Work out the finished part from the listing and answer in its coordinate system (mm). A direction names the side the tool comes from. Coordinates: 2 decimals unless noted, no trailing zeros. Order: outer loops, then holes, each group sorted by start corner. A loop starts at its lowest first (then second) coordinate and runs counter-clockwise, first axis right, second up. Notation, with made-up numbers: M 40.5,46 L 64.5,46 A13 cw 64.5,60 Z; hole C 74.25,-26.5 d7. An arc over 180 degrees is marked long. Use a Markdown table: item, result. Add a question column.
from build123d import *

# Parameters (mm, degrees)
F1_DEPTH  = 3
F2_R      = 1.5
F3_DEPTH  = 25
F5_DEPTH  = 3
F7_D      = 3
F7_DEPTH  = 3
F7_TIP    = 0.9012909285
F8_DEPTH  = 3
F9_R      = 1.5
F9_R_2    = 4
F10_DEPTH = 25


# Not quite as in the source:
# - a feature names something its author has since deleted; it is built from what else it names


with BuildPart() as f1:
    # F0 (on Front) → F1 (new body)
    with BuildSketch(Plane.XZ):
        with BuildLine():
            Line((-75, -60), (75, -60))
            ThreePointArc((75, -60), (78.5355339059, -58.5355339059), (80, -55))
            Line((80, -55), (80, 55))
            ThreePointArc((80, 55), (78.5355339059, 58.5355339059), (75, 60))
            Line((75, 60), (-75, 60))
            ThreePointArc((-75, 60), (-78.5355339059, 58.5355339059), (-80, 55))
            Line((-80, 55), (-80, -55))
            ThreePointArc((-80, -55), (-78.5355339059, -58.5355339059), (-75, -60))
        make_face()
    extrude(amount=F1_DEPTH)

    # F2 (on Front) → F3 (cut)
    with BuildSketch(Plane.XZ):
        with Locations((-75, 55)):
            Circle(F2_R)
        with Locations((75, 55)):
            Circle(F2_R)
        with Locations((75, -55)):
            Circle(F2_R)
        with Locations((-75, -55)):
            Circle(F2_R)
    extrude(amount=F3_DEPTH, mode=Mode.SUBTRACT)

    # F4 (on face) → F5 (cut)
    with BuildSketch(Plane.XZ.offset(3)):
        with BuildLine():
            ThreePointArc((72.5, 47.5), (71.0355339059, 51.0355339059), (67.5, 52.5))
            Line((67.5, 52.5), (54.75, 52.5))
            Line((54.75, 52.5), (54.75, 60))
            Line((54.75, 60), (-1.25, 60))
            Line((-1.25, 60), (-1.25, 52.5))
            Line((-1.25, 52.5), (-34, 52.5))
            ThreePointArc((-34, 52.5), (-34.7071067812, 52.2071067812), (-35, 51.5))
            Line((-35, 51.5), (-35, 15))
            ThreePointArc((-35, 15), (-34.7071067812, 14.2928932188), (-34, 14))
            Line((-34, 14), (-17, 14))
            ThreePointArc((-17, 14), (-16.2928932188, 13.7071067812), (-16, 13))
            Line((-16, 13), (-16, -51.5))
            ThreePointArc((-16, -51.5), (-15.7071067812, -52.2071067812), (-15, -52.5))
            Line((-15, -52.5), (67.5, -52.5))
            ThreePointArc((67.5, -52.5), (71.0355339059, -51.0355339059), (72.5, -47.5))
            Line((72.5, -47.5), (72.5, 47.5))
        make_face()
    extrude(amount=-F5_DEPTH, mode=Mode.SUBTRACT)

    # F7
    with Locations(Plane.XZ.offset(3)):
        with Locations((-56, 56), (-39, 56)):
            Hole(F7_D / 2, depth=F7_DEPTH)
            with Locations((0, 0, -(F7_DEPTH + F7_TIP / 2))):  # 118° drill point
                Cone(0, F7_D / 2, F7_TIP, mode=Mode.SUBTRACT)

    # F4 (on face) → F8 (cut)
    with BuildSketch(Plane.XZ.offset(3)):
        with BuildLine():
            ThreePointArc((72.5, 47.5), (71.0355339059, 51.0355339059), (67.5, 52.5))
            Line((67.5, 52.5), (54.75, 52.5))
            Line((54.75, 52.5), (54.75, 60))
            Line((54.75, 60), (-1.25, 60))
            Line((-1.25, 60), (-1.25, 52.5))
            Line((-1.25, 52.5), (-34, 52.5))
            ThreePointArc((-34, 52.5), (-34.7071067812, 52.2071067812), (-35, 51.5))
            Line((-35, 51.5), (-35, 15))
            ThreePointArc((-35, 15), (-34.7071067812, 14.2928932188), (-34, 14))
            Line((-34, 14), (-17, 14))
            ThreePointArc((-17, 14), (-16.2928932188, 13.7071067812), (-16, 13))
            Line((-16, 13), (-16, -51.5))
            ThreePointArc((-16, -51.5), (-15.7071067812, -52.2071067812), (-15, -52.5))
            Line((-15, -52.5), (67.5, -52.5))
            ThreePointArc((67.5, -52.5), (71.0355339059, -51.0355339059), (72.5, -47.5))
            Line((72.5, -47.5), (72.5, 47.5))
        make_face()
        with BuildLine():
            ThreePointArc((-67.5, 52.5), (-71.0355339059, 51.0355339059), (-72.5, 47.5))
            Line((-72.5, 47.5), (-72.5, 15))
            ThreePointArc((-72.5, 15), (-72.2071067812, 14.2928932188), (-71.5, 14))
            Line((-71.5, 14), (-61, 14))
            ThreePointArc((-61, 14), (-60.2928932188, 14.2928932188), (-60, 15))
            Line((-60, 15), (-60, 51.5))
            ThreePointArc((-60, 51.5), (-60.2928932188, 52.2071067812), (-61, 52.5))
            Line((-61, 52.5), (-67.5, 52.5))
        make_face()
    extrude(amount=-F8_DEPTH, mode=Mode.SUBTRACT)

    # F9 (on face) → F10 (cut)
    with BuildSketch(Plane.XZ.offset(3)):
        with Locations((-70, 9)):
            Circle(F9_R)
        with Locations((-60, -45)):
            Circle(F9_R_2)
        with Locations((-70, -32)):
            Circle(F9_R)
    extrude(amount=-F10_DEPTH, mode=Mode.SUBTRACT)


solid = f1.part
(1) Straight lines are drawn through the part: line 1 (Z direction, x = 75, y = -0.8); line 2 (X direction, y = -2.5, z = 38.5); line 3 (X direction, y = -1.45, z = -55). For each, find the intervals that lie inside material, in ascending order.
(2) A cutting plane is placed at A-A on z = -26.5. Write down the section's boundary in (x, y).
(3) Which of the six approach directions +Z, -Z, +X, -X, +Y, -Y give full straight-line access (tool end or side, diameter ignored) to faces 4 (the cylindrical face through (-79, -1, -58)), 5 (the cylindrical face through (-71, -1.52, 51.07))?
(4) A cutting plane is placed at D-D on y = -1.3. Count the separate pieces of the cut face and the enclosed holes in it, plus the area to 3 significant figures.
(5) The mould has two halves that part along Z. Classify faces 1 (the cylindrical face through (79, -1, 58)), 2 (the cylindrical face through (-56.185, -1.521, -43.799)), 3 (the cylindrical face through (78, -1, -59)): pulls with the +Z half, pulls with the -Z half, needs draft (parallel to the pull), parting line crosses it, or undercut.
(6) Given P1, Ø5, axis at x = -70, z = 9, coming from the +Y side; P2, Ø1.5, axis at x = 38, y = -1.5, coming from the +Z side; P3, Ø1.5, axis at y = -1.5, z = 56, coming from the +X side, each flat-ended and moving along its own axis, determine where each tip first touches the part or whether it passes through.
(7) A cutting plane is placed at C-C on z = -45. Write down the section's boundary in (x, y), plus the area to 4 significant figures.
(8) A cutting plane is placed at B-B on x = 60.5. Write down the section's boundary in (y, z), plus the area to 3 significant figures.
From the geometry:
| question | item | result |
|---|---|---|
| 1 | line 1 | z = -60 to -56.5, -53.5 to 53.5, 56.5 to 60 |
| 1 | line 2 | x = -80 to -72.5, -60 to -35, 72.5 to 80 |
| 1 | line 3 | x = -80 to -76.5, -73.5 to 73.5, 76.5 to 80 |
| 2 | outline | M -80,-3 L -16,-3 L -16,0 L -80,0 Z; M 72.5,-3 L 80,-3 L 80,0 L 72.5,0 Z |
| 3 | face 4 | -Z, -X, +Y, -Y |
| 3 | face 5 | +Y, -Y |
| 4 | separate pieces | 1 |
| 4 | enclosed holes | 10 |
| 4 | area | 8,160 mm2 |
| 5 | face 1 | pulls with the +Z half |
| 5 | face 2 | undercut |
| 5 | face 3 | pulls with the -Z half |
| 6 | P1 | stops at y = 0 |
| 6 | P2 | stops at z = -52.5 |
| 6 | P3 | stops at x = 79.99 |
| 7 | outline | M -80,-3 L -64,-3 L -64,0 L -80,0 Z; M -56,-3 L -16,-3 L -16,0 L -56,0 Z; M 72.5,-3 L 80,-3 L 80,0 L 72.5,0 Z |
| 7 | area | 190.5 mm2 |
| 8 | outline | M -3,-60 L 0,-60 L 0,-52.5 L -3,-52.5 Z; M -3,52.5 L 0,52.5 L 0,60 L -3,60 Z |
| 8 | area | 45.0 mm2 |
